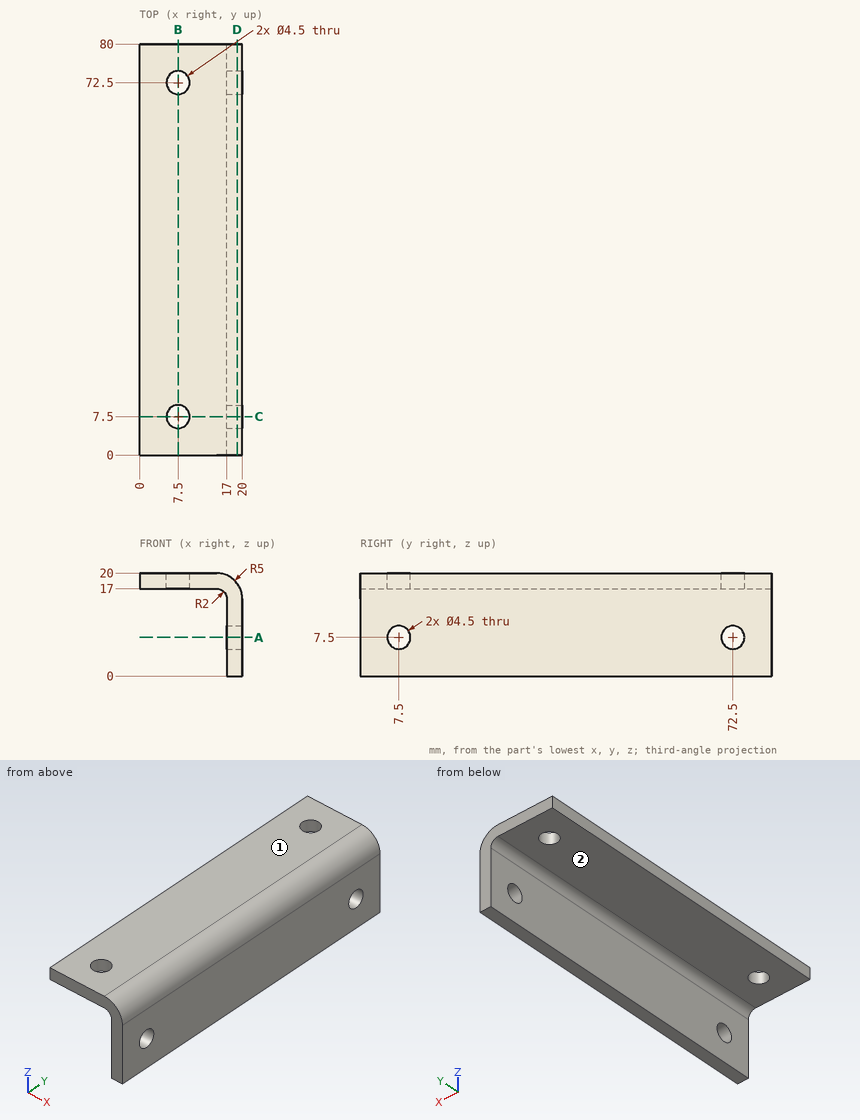
For this review, use the dimensioned drawing (mm, ordinates from the lowest corner) and the shaded views. A direction names the side the tool comes from. Coordinates: 2 decimals unless noted, no trailing zeros. Loops run counter-clockwise (first coordinate to the right, second up) from the corner with the lowest first, then second, coordinate; pieces in that order, holes last. Notation, with made-up numbers: M 69.5,24 L 106.5,24 A22 cw 106.5,37 Z; hole C 18.25,79 d7. An arc over 180 degrees is marked long. Answer as CSV lines item,"result".
Item 1: For P1, Ø4, axis at y = 21.5, z = 5, coming from the -X side; P2, Ø10, axis at x = 11, y = 21, coming from the -Z side; P3, Ø4, axis at x = 13, y = 42, coming from the -Z side; P4, Ø6, axis at y = 65, z = 18, coming from the -X side, all flat-tipped, find the tip position at first contact; note any pin that passes through.
Answer list:
P1,"x = 17"
P2,"z = 16.73"
P3,"z = 17"
P4,"x = 0"
Item 2: Add section D-D on x = 19. State the section outline as (y, z) points.
Answer list:
outline,"M 0,0 L 80,0 L 80,18 L 0,18 Z; hole C 7.5,7.5 d4.5; hole C 72.5,7.5 d4.5"
Item 3: For probe 1 along Y at (x, z) = (7.5, 19.1); probe 2 along X at (y, z) = (52.5, 3.75), list the stretches that pass through material, from the lowest coordinate up.
Answer list:
probe 1,"0 to 5.25, 9.75 to 70.25, 74.75 to 80"
probe 2,"17 to 20"
Item 4: Machinability: for the marked faces 1 and 2, which of the approach directions +Z, -Z, +X, -X, +Y, -Y give a long, thin tool a straight path to every point of the face, cutting with its end or side? Answer none if there is none.
Answer list:
face 1,"+Z, +X, -X, +Y, -Y"
face 2,"-Z, -X, +Y, -Y"
Item 5: Add section C-C on y = 7.5. State the section outline as (x, z) points, plus the area to 3 significant figures.
Answer list:
outline,"M 0,17 L 5.25,17 L 5.25,20 L 0,20 Z; M 9.75,17 L 15,17 A2 cw 17,15 L 17,9.75 L 20,9.75 L 20,15 A5 ccw 15,20 L 9.75,20 Z; M 17,0 L 20,0 L 20,5.25 L 17,5.25 Z"
area,"79.5 mm²"
Item 6: Add section A-A on z = 7.5. State the section outline as (x, y) points, plus the area to 3 significant figures.
Answer list:
outline,"M 17,0 L 20,0 L 20,5.25 L 17,5.25 Z; M 17,9.75 L 20,9.75 L 20,70.25 L 17,70.25 Z; M 17,74.75 L 20,74.75 L 20,80 L 17,80 Z"
area,"213 mm²"
Item 7: Add section B-B on x = 7.5. State the section outline as (y, z) points, plus the area to 3 significant figures.
Answer list:
outline,"M 0,17 L 5.25,17 L 5.25,20 L 0,20 Z; M 9.75,17 L 70.25,17 L 70.25,20 L 9.75,20 Z; M 74.75,17 L 80,17 L 80,20 L 74.75,20 Z"
area,"213 mm²"
